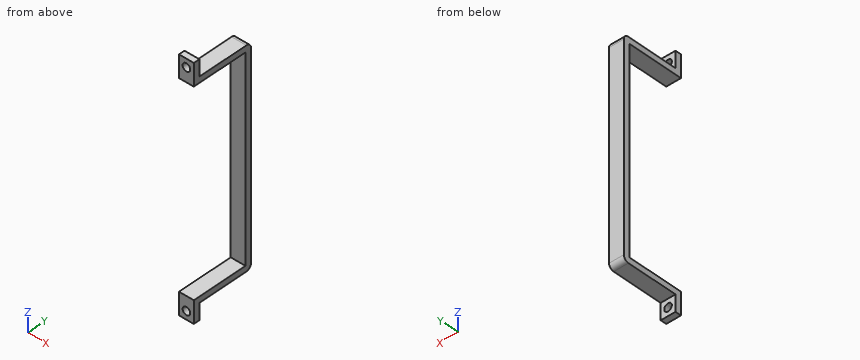
Autodesk Inventor part; units mm, degrees
ref_plane "YZ Plane" through (0, 0, 0) normal (1, 0, 0) x (0, 1, 0)
ref_plane "XZ Plane" through (0, 0, 0) normal (0, 1, 0) x (-1, 0, 0)
ref_plane "XY Plane" through (0, 0, 0) normal (0, 0, 1) x (1, 0, 0)
sketch "Sketch1" plane through (0, 0, 0) normal (1, 0, 0) x (0, 1, 0)
  line L0 (0, 0) -> (0, -80.85)
  line L1 (0, 0) -> (-22.5, 0)
  line L2 (-22.5, 0) -> (-22.5, 9)
  line L3 (-22.5, 9) -> (-20.1, 9)
  line L4 (-20.1, 9) -> (-20.1, 2.4)
  line L5 (-20.1, 2.4) -> (2.4, 2.4)
  line L6 (2.4, 2.4) -> (2.4, -40.425)
  line L7 (0, -80.85) -> (-22.5, -80.85)
  line L8 (-22.5, -80.85) -> (-22.5, -89.85)
  line L9 (-22.5, -89.85) -> (-20.1, -89.85)
  line L10 (-20.1, -89.85) -> (-20.1, -83.25)
  line L11 (-20.1, -83.25) -> (2.4, -83.25)
  line L12 (2.4, -83.25) -> (2.4, -40.425)
  dimension "d0" = 80.85
  dimension "d17" = 22.5
  dimension "d18" = 9
  dimension "d19" = 2.4
  dimension "d20" = 6.6
  dimension "d21" = 22.5
  dimension "d23" = 2.4
  dimension "d24" = 2.4
  dimension "d25" = 9
  dimension "d26" = 2.4
extrude "Extrusion1" add sketch "Sketch1" along normal blind 6
fillet "Fillet1" radius 2 1 edges at (3, 2.4, 2.4)
fillet "Fillet2" radius 2 1 edges at (3, 2.4, -83.25)
sketch "Sketch3" plane through (0, -20.1, 9) normal (0, 1, 0) x (1, 0, 0)
  line L0 (0, 6.6) -> (0, 0)
  line L1 (0, 6.6) -> (6, 6.6)
  circle A0 centre (3, 3.3) radius 1.55
  line L2 (0, 92.25) -> (6, 92.25)
  line L3 (6, 98.85) -> (6, 92.25)
  circle A1 centre (3, 95.55) radius 1.55
  line L4 (0, 0) -> (6, 0)
  line L5 (0, 98.85) -> (0, 92.25)
  point P0 (0, 9)
  dimension "d29" = 3.1
  dimension "d30" = 3.1
extrude "Extrusion3" cut sketch "Sketch3" against normal blind 10
properties part number "battery_pack_clamp" material "PET Plastic"
Geometry: final body of the model. Coordinates: model frame, mm. Give positions to 0.01 mm unless a question says otherwise; leave off trailing zeros. Write each loop counter-clockwise with the first axis right and the second up, starting at its lowest first coordinate (ties: lowest second). Pieces come first, ordered by that corner, then holes. Notation, with made-up numbers: (12.5, 29.25) -> (25.5, 29.25) arc R22 ccw to (25.5, 43.25) -> close; hole circle Ø7 at (1, 69.5). An arc over 180 degrees is marked (long way). Answer as a JSON object with one key per item and string values.
1. Cut plane A-A on z = 5.7. Output: boundary loops of the cut face in (x, y), and give its area (3 significant figures).
Ans:
{"outline": "(0, -22.5) -> (1.45, -22.5) -> (1.45, -20.1) -> (0, -20.1) -> close; (4.55, -22.5) -> (6, -22.5) -> (6, -20.1) -> (4.55, -20.1) -> close", "area": "6.96 mm^2"}
2. Contact query for flat-ended pins moving along their axis: pin 1 (2.5 mm diameter, centred on x = 3, z = -86.55, fed in from -Y); pin 2 (3 mm diameter, centred on x = 2, y = -10.5, fed in from -Z); pin 3 (1.8 mm diameter, centred on x = 2.5, z = -85.5, fed in from +Y). Output: stop coordinate, or through.
Ans:
{"pin 1": "passes through", "pin 2": "stops at z = -83.25", "pin 3": "stops at y = -20.1"}
3. Cut plane C-C on x = 3. Output: boundary loops of the cut face in (y, z), and give its area (3 significant figures).
Ans:
{"outline": "(-22.5, -89.85) -> (-20.1, -89.85) -> (-20.1, -88.1) -> (-22.5, -88.1) -> close; (-22.5, -85) -> (-20.1, -85) -> (-20.1, -83.25) -> (0.4, -83.25) arc R2 ccw to (2.4, -81.25) -> (2.4, 0.4) arc R2 ccw to (0.4, 2.4) -> (-20.1, 2.4) -> (-20.1, 4.15) -> (-22.5, 4.15) -> (-22.5, 0) -> (0, 0) -> (0, -80.85) -> (-22.5, -80.85) -> close; (-22.5, 7.25) -> (-20.1, 7.25) -> (-20.1, 9) -> (-22.5, 9) -> close", "area": "329 mm^2"}
4. Cut plane D-D on z = -42. Output: boundary loops of the cut face in (x, y), and give its area (3 significant figures).
Ans:
{"outline": "(0, 0) -> (6, 0) -> (6, 2.4) -> (0, 2.4) -> close", "area": "14.4 mm^2"}
5. Ray query, probe 1 along Z at (x, y) = (3, -21.75); probe 2 along Z at (x, y) = (1.6, -11.5); probe 3 along Z at (x, y) = (3.85, -21). Return the intervals inside material, ascending. Write a range as from..to.
Ans:
{"probe 1": "z = -89.85..-88.1, -85..-80.85, 0..4.15, 7.25..9", "probe 2": "z = -83.25..-80.85, 0..2.4", "probe 3": "z = -89.85..-87.85, -85.25..-80.85, 0..4.4, 7..9"}
6. Cut plane B-B on y = -1.5. Output: boundary loops of the cut face in (x, z).
Ans:
{"outline": "(0, -83.25) -> (6, -83.25) -> (6, -80.85) -> (0, -80.85) -> close; (0, 0) -> (6, 0) -> (6, 2.4) -> (0, 2.4) -> close"}
